Can you work these out from the model? Positions are in its coordinate system, mm. Coordinates: 2 decimals unless noted, no trailing zeros. Loops run counter-clockwise (first coordinate to the right, second up) from the corner with the lowest first, then second, coordinate; pieces in that order, holes last. Notation, with made-up numbers: (31.5, 53.5) -> (75.5, 53.5) arc R24 ccw to (75.5, 82.5) -> close; hole circle Ø6 at (12.5, 70). An arc over 180 degrees is marked (long way). Put each result on its own line as item: value. Start each with the question number.
Item 1: If we section it at D-D on z = 0.65: State how many separate pieces and enclosed holes the cut face has, plus the area to 3 significant figures.
Item 2: Please list where these lines run through material, in increasing order: L1, parallel to Y at x = 33, z = 1.15; L2, parallel to Y at x = 46.5, z = 0.6; L3, parallel to X at y = 48, z = 0.15. Write a range as from..to.
Item 3: If we section it at A-A on y = 0: Please give me the cut outline in (x, z), plus the area to 3 significant figures.
Item 4: If we section it at B-B on x = -30: Please give me the cut outline in (y, z).
Item 5: If we section it at C-C on y = -16: Please give me the cut outline in (x, z), plus the area to 3 significant figures.
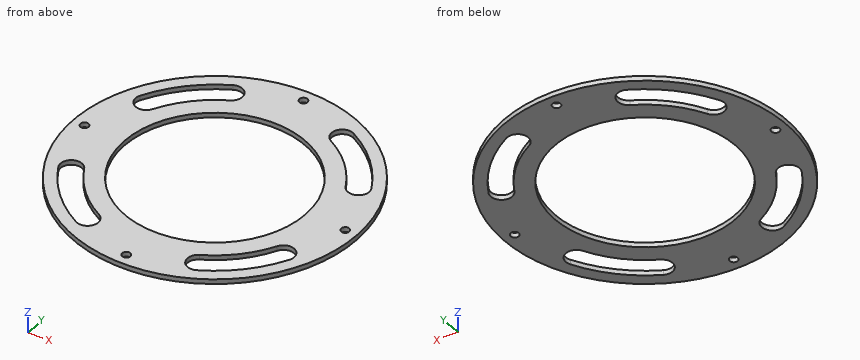
```python
from build123d import *

# Parameters (mm, degrees)
SKETCH_1_R               = 59.5
SKETCH_1_R_2             = 1.7
EXTRUDE_4_DEPTH          = 2
SKETCH_2_R               = 38
CUT_EXTRUDE_1_DEPTH      = 2
CUT_EXTRUDE_3_DEPTH      = 2
PATTERN_CIRCULAR_2_COUNT = 4


with BuildPart() as part:
    # 草图1 → 凸台-拉伸4 (new body)
    with BuildSketch(Plane.XY):
        Circle(SKETCH_1_R)
        with Locations((0, 54.5)):
            Circle(SKETCH_1_R_2, mode=Mode.SUBTRACT)
        with Locations((54.5, 0)):
            Circle(SKETCH_1_R_2, mode=Mode.SUBTRACT)
        with Locations((0, -54.5)):
            Circle(SKETCH_1_R_2, mode=Mode.SUBTRACT)
        with Locations((-54.5, 0)):
            Circle(SKETCH_1_R_2, mode=Mode.SUBTRACT)
    extrude(amount=EXTRUDE_4_DEPTH)

    # 草图2 → 切除-拉伸1 (cut)
    with BuildSketch(Plane.XY.offset(2)):
        Circle(SKETCH_2_R)
    extrude(amount=-CUT_EXTRUDE_1_DEPTH, mode=Mode.SUBTRACT)

    # 草图4 → 切除-拉伸3 (cut)
    with BuildSketch(Plane.XY.offset(2)):
        with BuildLine():
            ThreePointArc((21.039420393, 40.34343552), (32.173358544, 32.173358544), (40.34343552, 21.039420393))
            ThreePointArc((40.34343552, 21.039420393), (46.414267423, 19.130232084), (48.323455732, 25.201063987))
            ThreePointArc((48.323455732, 25.201063987), (38.537319575, 38.537319575), (25.201063987, 48.323455732))
            ThreePointArc((25.201063987, 48.323455732), (19.130232084, 46.414267423), (21.039420393, 40.34343552))
        make_face()
    cut_extrude_3 = extrude(amount=-CUT_EXTRUDE_3_DEPTH, mode=Mode.SUBTRACT)

    # 阵列(圆周)2: 切除-拉伸3 ×4 about axis
    pattern_circular_2_axis = Axis((0, 0, 0), (0, 0, 1))
    for i in range(1, PATTERN_CIRCULAR_2_COUNT):
        add(cut_extrude_3.rotate(pattern_circular_2_axis, i * 360 / PATTERN_CIRCULAR_2_COUNT), mode=Mode.SUBTRACT)


solid = part.part
```
Solutions:
1. separate pieces: 1
1. enclosed holes: 9
1. area: 5,200 mm^2
2. L1: -49.51..-43.37, -31.32..-18.84, 18.84..31.32, 43.37..49.51
2. L2: -37.12..-28.43, -19.18..19.18, 28.43..37.12
2. L3: -35.16..-25.81, -20.51..20.51, 25.81..35.16
3. outline: (-59.5, 0) -> (-56.2, 0) -> (-56.2, 2) -> (-59.5, 2) -> close; (-52.8, 0) -> (-38, 0) -> (-38, 2) -> (-52.8, 2) -> close; (38, 0) -> (52.8, 0) -> (52.8, 2) -> (38, 2) -> close; (56.2, 0) -> (59.5, 0) -> (59.5, 2) -> (56.2, 2) -> close
3. area: 72.4 mm^2
4. outline: (-51.38, 0) -> (-45.5, 0) -> (-45.5, 2) -> (-51.38, 2) -> close; (-34.21, 0) -> (-23.32, 0) -> (-23.32, 2) -> (-34.21, 2) -> close; (23.32, 0) -> (34.21, 0) -> (34.21, 2) -> (23.32, 2) -> close; (45.5, 0) -> (51.38, 0) -> (51.38, 2) -> (45.5, 2) -> close
5. outline: (-57.31, 0) -> (-34.47, 0) -> (-34.47, 2) -> (-57.31, 2) -> close; (34.47, 0) -> (57.31, 0) -> (57.31, 2) -> (34.47, 2) -> close
5. area: 91.4 mm^2
